Verification items for the finished model (mm, model axes). A direction names the side the tool comes from. Round coordinates to 2 decimals unless told otherwise and drop trailing zeros. Loops run counter-clockwise (first coordinate to the right, second up) from the corner with the lowest first, then second, coordinate; pieces in that order, holes last.
from build123d import *

# Parameters (mm, degrees)
F0_R     = 28.575
F1_DEPTH = 12.7
F2_DEPTH = 6.35


with BuildPart() as f1:
    # F0 (on Right) → F1 (new body)
    with BuildSketch(Plane.YZ):
        Polygon((-76.2, -25.46159), (-25.4, -76.13841), (25.4, -76.13841), (76.2, -25.46159), (76.2, 76.13841), (-76.2, 76.13841), align=None)
        Circle(F0_R, mode=Mode.SUBTRACT)
    extrude(amount=F1_DEPTH)

    # F0 (on Right) → F2 (join)
    with BuildSketch(Plane.YZ):
        Polygon((89.998516, 89.934262), (77.298516, 89.934262), (-77.298516, 90.057443), (-89.998516, 90.057443), (-89.998516, -29.635283), (-31.75, -87.742557), (31.75, -87.742557), (89.998516, -29.635283), (89.998516, 77.234262), align=None)
        Polygon((25.4, -76.13841), (-25.4, -76.13841), (-76.2, -25.46159), (-76.2, 76.13841), (76.2, 76.13841), (76.2, -25.46159), align=None, mode=Mode.SUBTRACT)
    extrude(amount=F2_DEPTH)


solid = f1.part
1. Tool access check on faces 1 (the face through (9, 76.2, 25)), 2 (the face through (9.5, 50.4, -51.2)), 3 (the face through (9.5, -51.2, -50.4)), 4 (the face through (9, 1, 76.138)). Record the directions out of +Z, -Z, +X, -X, +Y, -Y that give a thin tool (end or side, any length) a straight path to the whole face; none if there is none.
2. Release check for a two-part mould opening along Y. For faces 5 (the face through (3, 89.999, 29)), 6 (the face through (6.261, -28.547, 1.256)), 7 (the face through (9, -76.2, 26)), 8 (the face through (9, 0, -76.138)) record: released by +Y, released by -Y, zero draft, split by the parting line, or undercut.
3. Scan lines: L1, parallel to Z at x = 8.75, y = 0 (3 decimals); L2, parallel to Z at x = 6.25, y = 0 (3 decimals); L3, parallel to Y at x = 5.5, z = -25. Record each from-to range of solid material in increasing order.
4. Section check A-A (z = 0). Enter the section's corners in (x, y) (3 decimals).
5. Section check D-D (z = 38). Enter the section's corners in (x, y), then the cut area to 3 significant figures.
6. Section check C-C (y = 15.5). Enter the section's corners in (x, z).
7. Section check B-B (x = 9.75). Enter the section's corners in (y, z) (3 decimals), then the cut area to 3 significant figures.
8. Gauge pin test, flat ends, axial feed: P1, Ø7, axis at x = 8, y = 34, coming from the +Z side; P2, Ø2, axis at x = 5.5, y = -69, coming from the +Z side; P3, Ø5, axis at x = 10.5, z = 31, coming from the +Y side. Record the tip position at first contact, or that the pin passes through.
Taken from the geometry:
1. face 1: +Z, -Z, +X, +Y
1. face 2: -Z, +X, +Y
1. face 3: -Z, +X, -Y
1. face 4: +Z, +X, +Y, -Y
2. face 5: released by +Y
2. face 6: undercut
2. face 7: released by -Y
2. face 8: zero draft
3. L1: z = -76.138 to -28.575, 28.575 to 76.138
3. L2: z = -87.743 to -28.575, 28.575 to 89.996
3. L3: y = -90 to -13.84, 13.84 to 90
4. outline: (0, -89.999) - (6.35, -89.999) - (6.35, -76.2) - (12.7, -76.2) - (12.7, -28.575) - (0, -28.575) - close; (0, 28.575) - (12.7, 28.575) - (12.7, 76.2) - (6.35, 76.2) - (6.35, 89.999) - (0, 89.999) - close
5. outline: (0, -90) - (6.35, -90) - (6.35, -76.2) - (12.7, -76.2) - (12.7, 76.2) - (6.35, 76.2) - (6.35, 90) - (0, 90) - close
5. area: 2,110 mm2
6. outline: (0, -87.74) - (6.35, -87.74) - (6.35, -76.14) - (12.7, -76.14) - (12.7, -24.01) - (0, -24.01) - close; (0, 24.01) - (12.7, 24.01) - (12.7, 76.14) - (6.35, 76.14) - (6.35, 89.98) - (0, 89.98) - close
7. outline: (-76.2, -25.462) - (-25.4, -76.138) - (25.4, -76.138) - (76.2, -25.462) - (76.2, 76.138) - (-76.2, 76.138) - close; hole circle Ø57.15 at (0, 0)
7. area: 18,100 mm2
8. P1: stops at z = 89.97
8. P2: stops at z = 90.05
8. P3: stops at y = 76.2
